Input: part model. Units: mm. Frame: model coordinates. A direction names the side the tool comes from. Give positions to 0.01 mm unless a question says otherwise; leave off trailing zeros. Loops run counter-clockwise (first coordinate to the right, second up) from the corner with the lowest first, then second, coordinate; pieces in that order, holes last. Notation, with made-up numbers: (12.25, 26) - (69.25, 26) arc R19 ccw to (69.25, 31) - close; hole circle Ø10 at (58, -24.75). An arc over 180 degrees is marked (long way). Answer as a JSON object with one key per item and string values. Group by question number.
(1) Mould query, pull axis Z, two halves, no side actions, for faces 1 (the flat face through (0, 2, 4)), 2 (the conical face through (-6.2, 0.99, -1.69)), 3 (the flat face through (8.9, 3, -2)). Classes: +Z half, -Z half, draft (parallel to the pull), parting line (faces both ways), or undercut.
(2) Section query A-A (y = 3.25). Return loops of the section in (x, z), plus the area to 3 significant figures.
(3) Section query B-B (y = 18.25). Return loops of the section in (x, z), plus the area to 3 significant figures.
(4) Material intervals for L1, parallel to Y at x = 3.75, z = 1.5; L2, parallel to X at y = 5.75, z = -2.75; L3, parallel to X at y = 7.75, z = -2, sorted ascending.
(5) Pin query (flat end, axial travel): P1, Ø1.5, axis at x = -3, y = 8, coming from the +Z side; P2, Ø4, axis at x = 6.5, z = 0.5, coming from the +Y side; P3, Ø2, axis at x = -2, z = 2.5, coming from the +Y side; P4, Ø4, axis at x = -4, y = 16.5, coming from the -Z side. Return the tip coordinate at first contact, or that it passes through.
(6) Access query for faces 4 (the flat face through (-3, 5.5, 3)), 5 (the flat face through (3, 5.5, -3)), 6 (the flat face through (-4, 5, 2)), 7 (the flat face through (4, 5, -2)). Directions: +Z, -Z, +X, -X, +Y, -Y. A direction counts if a zero-diameter tool reaches every point of the face in a straight line with its end or side. Return the directions, or none.
```python
from build123d import *

# Parameters (mm, degrees)
EXTRUDE_1_DEPTH     = 4
CUT_EXTRUDE_1_DEPTH = 1.5
SKETCH_2_R          = 4
EXTRUDE_2_DEPTH     = 16
CUT_EXTRUDE_2_DEPTH = 5
CHAMFER_2_SIZE      = 1


with BuildPart() as part:
    # Эскиз1 → Бобышка-Вытянуть1 (new body, symmetric)
    with BuildSketch(Plane.XY):
        Polygon((8.9, 0), (-8.9, 0), (-8.9, 4), (-4, 4), (-4, 5.5), (4, 5.5), (4, 4), (8.9, 4), align=None)
    extrude(amount=EXTRUDE_1_DEPTH, both=True)

    # Эскиз3 → Вырез-Вытянуть1 (cut)
    with BuildSketch(Plane(origin=(0, 5.5, 0), x_dir=(1, 0, 0), z_dir=(0, 1, 0))):
        with BuildLine():
            Line((-4, 0), (-4, 4))
            Line((-4, 4), (0, 4))
            ThreePointArc((0, 4), (-2.828427125, 2.828427125), (-4, 0))
        make_face()
        with BuildLine():
            Line((0, -4), (4, -4))
            Line((4, -4), (4, 0))
            ThreePointArc((4, 0), (2.828427125, -2.828427125), (0, -4))
        make_face()
    extrude(amount=-CUT_EXTRUDE_1_DEPTH, mode=Mode.SUBTRACT)

    # Эскиз2 → Бобышка-Вытянуть2 (add)
    with BuildSketch(Plane(origin=(0, 5.5, 0), x_dir=(1, 0, 0), z_dir=(0, 1, 0))):
        with Locations(Location((0, 0, 0), (0, 0, 270))):  # turned: the seam where the file's is
            Circle(SKETCH_2_R)
    extrude(amount=EXTRUDE_2_DEPTH)

    # Эскиз4 → Вырез-Вытянуть2 (cut, through all)
    with BuildSketch(Plane(origin=(0, 4, 0), x_dir=(1, 0, 0), z_dir=(0, 1, 0))):
        with BuildLine():
            Line((-7.950471684, 4), (-8.9, 4))
            Line((-8.9, 4), (-8.9, 0))
            ThreePointArc((-8.9, 0), (-8.659364815, 2.055578022), (-7.950471684, 4))
        make_face()
        with BuildLine():
            Line((7.950471684, -4), (8.9, -4))
            Line((8.9, -4), (8.9, 0))
            ThreePointArc((8.9, 0), (8.659364815, -2.055578022), (7.950471684, -4))
        make_face()
    extrude(amount=-CUT_EXTRUDE_2_DEPTH, mode=Mode.SUBTRACT)

    # Вырез-По траектории1: sweep along a path in Эскиз6
    with BuildLine(Plane.XZ) as sweep_1_path:
        Line((0, -8.9), (8.9, -8.9))
        Line((8.9, -8.9), (8.9, 0))
        ThreePointArc((8.9, 0), (6.293250353, 6.293250353), (0, 8.9))
        Line((0, 8.9), (-8.9, 8.9))
        Line((-8.9, 8.9), (-8.9, 0))
        ThreePointArc((-8.9, 0), (-6.293250353, -6.293250353), (0, -8.9))
    # Эскиз5 → Вырез-По траектории1 (sweep, cut)
    with BuildSketch(Plane.XY.offset(4)):
        Polygon((-8.9, 2.5), (-4.8, 0), (-8.9, 0), align=None)
    sweep(path=sweep_1_path.line, transition=Transition.RIGHT, mode=Mode.SUBTRACT)

    # Фаска2
    chamfer_2_edges = [part.edges().sort_by_distance(p)[0] for p in [
        (0, 21.5, -4),
    ]]
    chamfer(chamfer_2_edges, length=CHAMFER_2_SIZE)


solid = part.part
```
Recorded:
{
 "1": {"face 1": "+Z half", "face 2": "-Z half", "face 3": "draft"},
 "2": {"outline": "(-8.9, 0) arc R8.9 ccw to (-7.95, -4) - (8.9, -4) - (8.9, 0) arc R8.9 ccw to (7.95, 4) - (-8.9, 4) - close", "area": "140 mm^2"},
 "3": {"outline": "circle Ø8 at (0, 0)", "area": "50.3 mm^2"},
 "4": {"L1": "y = 0 to 4", "L2": "x = -2.9 to 2.9", "L3": "x = -3.46 to 3.46"},
 "5": {"P1": "stops at z = 3.31", "P2": "stops at y = 4", "P3": "stops at y = 21.5", "P4": "stops at z = -3.46"},
 "6": {"face 4": "+Z, -X, +Y", "face 5": "-Z, +X, +Y", "face 6": "+Z, -Z, -X, +Y", "face 7": "+Z, -Z, +X, +Y"}
}
